Check sheet for the modelled part. Datum: model origin and axes. Units: mm. Face numbers are marked on the shaded views. Round coordinates to 2 decimals unless told otherwise and drop trailing zeros. Write each loop counter-clockwise with the first axis right and the second up, starting at its lowest first coordinate (ties: lowest second). Pieces come first, ordered by that corner, then holes. Notation, with made-up numbers: M 8.5,85 L 47.5,85 A34 cw 47.5,117 Z; hole C 4.25,10 d3. An arc over 180 degrees is marked long. Answer in a Markdown table with one row per item.
Autodesk Inventor part; units mm, degrees
ref_plane "Work Plane1" through (0, 0, 6.35) normal (0, 0, 1) x (1, 0, 0)
ref_plane "Work Plane4" through (0, 19.1494, 6.35) normal (-1, 0, 0) x (0, -1, 0)
ref_plane "YZ Plane" through (0, 0, 0) normal (1, 0, 0) x (0, 1, 0)
sketch "Sketch1" plane through (0, 0, 0) normal (0, 0, 1) x (1, 0, 0)
  circle A0 centre (0, 0) radius 16.51
  circle A1 centre (0, 0) radius 20.32
  dimension "d0" = 40.64
  dimension "d2" = 33.02
extrude "Extrusion1" add sketch "Sketch1" along normal blind 11.43
sketch "Sketch2" plane through (0, 0, 11.43) normal (0, 0, 1) x (1, 0, 0)
  circle A0 centre (0, 0) radius 20.32
  circle A1 centre (0, 0) radius 15.875
  dimension "d5" = 31.75
extrude "Extrusion2" add sketch "Sketch2" along normal blind 1.27
fillet "Fillet1" radius 0.508 1 edges at (-15.875, 0, 11.43)
fillet "Fillet2" radius 0.508 1 edges at (-15.875, 0, 12.7)
ref_plane "Work Plane1" through (0, 0, 6.35) normal (0, 0, 1) x (1, 0, 0)
sketch "Sketch3" plane through (0, 0, 6.35) normal (0, 0, 1) x (1, 0, 0)
  line L0 (-20.32, 19.1494) -> (-20.32, -22.3588)
  circle A0 centre (0, 0) radius 20.32
  dimension "d11" = 20.32
sketch "Sketch4" plane through (0, 0, 12.7) normal (0, 0, 1) x (1, 0, 0)
  circle A0 centre (0, 0) radius 20.32
  circle A1 centre (0, 0) radius 16.383
ref_plane "Work Plane3" through (-20.32, 19.1494, 6.35) normal (-1, 0, 0) x (0, -1, 0)
ref_plane "Work Plane2" through (0, 0, 12.7) normal (0, 0, 1) x (1, 0, 0)
ref_plane "Work Plane4" through (0, 19.1494, 6.35) normal (-1, 0, 0) x (0, -1, 0)
sketch "Sketch6" plane through (0, 19.1494, 6.35) normal (-1, 0, 0) x (0, -1, 0)
  line L0 (39.364, 6.35) -> (35.554, 6.35)
  arc A0 (35.554, 6.35) -> (20.314, 11.4045) centre (19.0928, -17.78) ccw
  line L1 (39.364, 6.35) -> (39.364, 6.35)
  line L2 (31.744, 13.97) -> (20.314, 13.97)
  line L3 (20.314, 13.97) -> (20.314, 11.4045)
  arc A1 (39.364, 6.35) -> (31.744, 13.97) centre (31.744, 6.35) ccw
  line L4 (39.4694, 6.35) -> (-1.1706, 6.35)
  line L5 (19.044, 13.97) -> (19.044, 8.477)
  point P0 (19.1494, -6.35)
  point P1 (19.044, 5.9584)
  point P2 (19.044, 27.5056)
  point P3 (19.044, 11.43)
  point P4 (39.364, 13.97)
  dimension "d24" = 3.81
  dimension "d25" = 20.32
  dimension "d26" = 5.08
  dimension "d27" = 29.21
  dimension "d28" = 7.62
  dimension "d29" = 7.62
  dimension "d30" = 0
revolve "Revolution1" add sketch "Sketch6" angle 360 about axis through (0, 0.1054, 20.32) along (0, 0, -1)
sketch "Sketch8" plane through (0, 0.1054, 20.32) normal (0, 0, 1) x (1, 0, 0)
  circle A0 centre (0, 0) radius 1.27
  point P0 (0, -0.1054)
extrude "Extrusion4" add sketch "Sketch8" against normal blind 2.5654
properties part number "Motor End Cap" material "PVC-Piping"
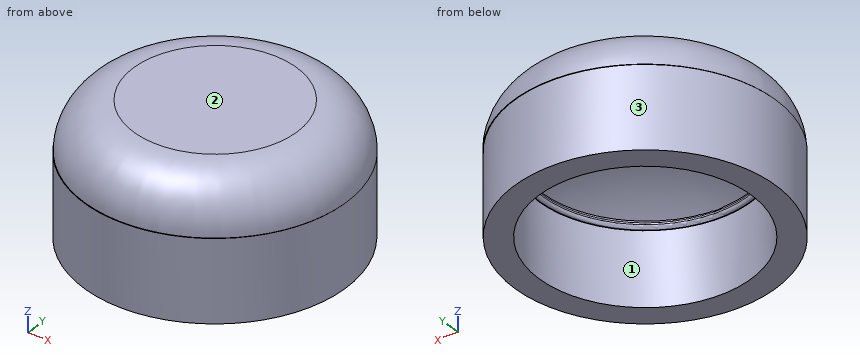
1. Section check B-B, the plane z = 19. Record the cut outline in (x, y).
Found:
| item | result |
|---|---|
| outline | C 0,0.11 d33.97 |
2. Section check A-A, the plane z = 1.75. Record the cut outline in (x, y), and give its area (3 significant figures).
Found:
| item | result |
|---|---|
| outline | C 0,0 d40.64; hole C 0,0 d33.02 |
| area | 441 mm2 |
3. Scan lines: L1, parallel to Y at x = 0, z = 12.1 (3 decimals); L2, parallel to X at y = -4, z = 2.25; L3, parallel to Y at x = 7, z = 1.5. Record each from-to range of solid material in increasing order.
Found:
| item | result |
|---|---|
| L1 | y = -20.32 to -15.875, 15.875 to 20.32 |
| L2 | x = -19.92 to -16.02, 16.02 to 19.92 |
| L3 | y = -19.08 to -14.95, 14.95 to 19.08 |
4. Go/stop test with flat-tipped pins: pin 1 (2 mm diameter, centred on x = 12, y = 13, fed in from +Z); pin 2 (19 mm diameter, centred on x = 0, y = 0, fed in from -Z); pin 3 (22.5 mm diameter, centred on x = 10, y = -15, fed in from +Z); pin 4 (12 mm diameter, centred on x = -3.5, z = 18, fed in from -Y). Record where each tip stops, or that it passes through.
Found:
| item | result |
|---|---|
| pin 1 | stops at z = 19.24 |
| pin 2 | stops at z = 16.17 |
| pin 3 | stops at z = 20.32 |
| pin 4 | stops at y = -20.31 |
5. Draft check along X on the marked faces 1, 2 and 3. Enter one of: +X half, -X half, draft (parallel to the pull), parting line (faces both ways), or undercut.
Found:
| item | result |
|---|---|
| face 1 | undercut |
| face 2 | draft |
| face 3 | parting line |
